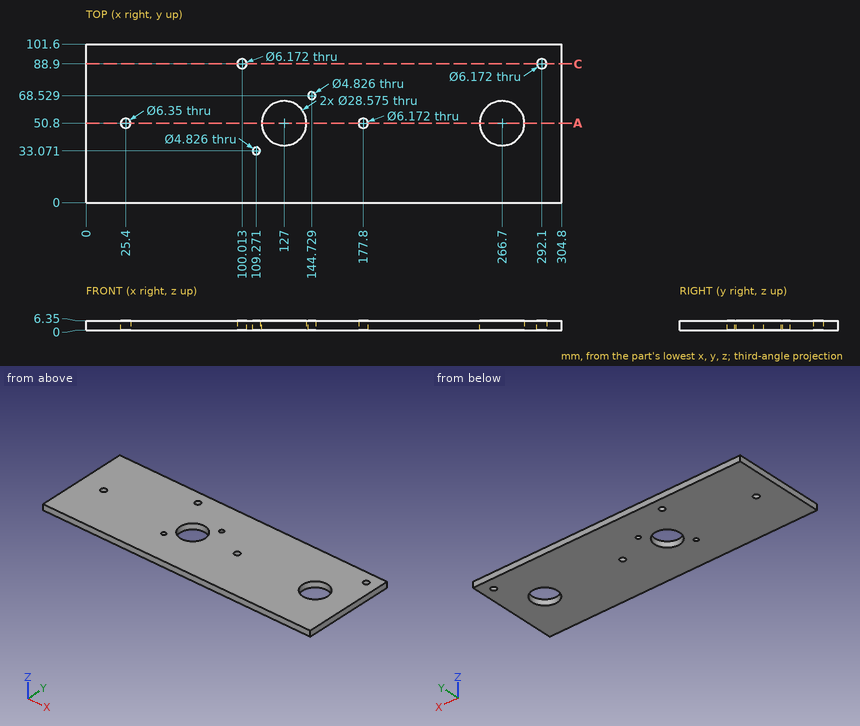
Check sheet for the drawn part. Datum: minimum x, y, z corner. Units: mm. Give positions to 0.01 mm unless a question says otherwise; leave off trailing zeros. Loops run counter-clockwise (first coordinate to the right, second up) from the corner with the lowest first, then second, coordinate; pieces in that order, holes last. Notation, with made-up numbers: M 51.5,52.5 L 81.5,52.5 A28 cw 81.5,80.5 Z; hole C 44.25,46.5 d5. An arc over 180 degrees is marked long. Return JSON: item names as keys, results as strings.
1) Section check A-A, the plane y = 50.8. Count the separate pieces of the cut face and the enclosed holes in it, and give its area (3 significant figures).
Findings:
{"separate pieces": "5", "enclosed holes": "0", "area": "1,490 mm2"}
2) Material ranges on L1, parallel to X at y = 89, z = 1.75 (1 decimal); L2, parallel to X at y = 52, z = 4.75 (1 decimal); L3, parallel to X at y = 62, z = 1.25, recorded low to high. Write a range as [from, to].
Findings:
{"L1": "x = [0, 96.9], [103.1, 289], [295.2, 304.8]", "L2": "x = [0, 22.5], [28.3, 112.8], [141.2, 175], [180.6, 252.5], [280.9, 304.8]", "L3": "x = [0, 118.13], [135.87, 257.83], [275.57, 304.8]"}
3) Section check C-C, the plane y = 88.9. Enter the section's corners in (x, z).
Findings:
{"outline": "M 0,0 L 96.93,0 L 96.93,6.35 L 0,6.35 Z; M 103.1,0 L 289.01,0 L 289.01,6.35 L 103.1,6.35 Z; M 295.19,0 L 304.8,0 L 304.8,6.35 L 295.19,6.35 Z"}
